from build123d import *

# Parameters (mm, degrees)
SKETCH1_W           = 8
SKETCH1_H           = 2
SKETCH1_W_2         = 2
SKETCH1_H_2         = 5
BOSS_EXTRUDE1_DEPTH = 2


with BuildPart() as part:
    # Sketch1 → Boss-Extrude1 (new body)
    with BuildSketch(Plane.XY):
        with BuildLine():
            Line((15.25, 3.5), (-15.25, 3.5))
            ThreePointArc((-15.25, 3.5), (-15.780330086, 3.280330086), (-16, 2.75))
            Line((-16, 2.75), (-16, -2.75))
            ThreePointArc((-16, -2.75), (-15.780330086, -3.280330086), (-15.25, -3.5))
            Line((-15.25, -3.5), (-3.5, -3.5))
            ThreePointArc((-3.5, -3.5), (-3.146446609, -3.646446609), (-3, -4))
            Line((-3, -4), (-3, -15.5))
            Line((-3, -15.5), (3, -15.5))
            Line((3, -15.5), (3, -4))
            ThreePointArc((3, -4), (3.146446609, -3.646446609), (3.5, -3.5))
            Line((3.5, -3.5), (15.25, -3.5))
            ThreePointArc((15.25, -3.5), (15.780330086, -3.280330086), (16, -2.75))
            Line((16, -2.75), (16, 2.75))
            ThreePointArc((16, 2.75), (15.780330086, 3.280330086), (15.25, 3.5))
        make_face()
        with Locations((-9, 0)):
            Rectangle(SKETCH1_W, SKETCH1_H, mode=Mode.SUBTRACT)
        with Locations((9, 0)):
            Rectangle(SKETCH1_W, SKETCH1_H, mode=Mode.SUBTRACT)
        with Locations((0, -11)):
            Rectangle(SKETCH1_W_2, SKETCH1_H_2, mode=Mode.SUBTRACT)
    extrude(amount=BOSS_EXTRUDE1_DEPTH)


solid = part.part
Here's how the part is built. I have some questions about the finished solid (model axes, mm). A direction names the side the tool comes from. Coordinates: 2 decimals unless noted, no trailing zeros. Order: outer loops, then holes, each group sorted by start corner. A loop starts at its lowest first (then second) coordinate and runs counter-clockwise, first axis right, second up. Notation, with made-up numbers: (-28, 2) - (-22, 2) arc R31 ccw to (-22, 35) - close; hole circle Ø5 at (-11, 52). An arc over 180 degrees is marked (long way). Use CSV: the item, a comma, the result in double quotes. Start each with the question number.
1. Suppose I cut it at B-B on z = 0.3. List the corners of the cut face in (x, y) for me, then the cut area to 3 significant figures.
2. Suppose I cut it at A-A on x = -9. List the corners of the cut face in (y, z) for me, then the cut area to 3 significant figures.
3. I'm going to push flat-ended pins straight in: pin 1 (1.5 mm diameter, centred on x = -9.5, y = 0, fed in from +Z); pin 2 (4 mm diameter, centred on x = 4, y = 0, fed in from -Z); pin 3 (0.6 mm diameter, centred on x = 8.5, z = 1, fed in from -Y). Where does each tip first touch, or does it pass through?
4. If we mould it in two halves opening along Y, with no side actions, what happens to faces 1 (the face through (0, 3.5, 1)), 2 (the face through (0, -3, 2)), 3 (the face through (-5, 0, 1))? For each: +Y half, -Y half, draft (parallel to the pull), parting line (faces both ways), or undercut.
5. For faces 4 (the face through (3, -10, 1)), 5 (the face through (-9, 1, 1)), 6 (the face through (-3, -10, 1)), which set-ups out of +Z, -Z, +X, -X, +Y, -Y let a thin tool reach every point of the face, with its end or its side?
6. Suppose I cut it at C-C on y = -14.25. List the corners of the cut face in (x, z) for me.
7. Suppose I cut it at D-D on x = 4. List the corners of the cut face in (y, z) for me.
8. Please list where these lines run through material, in increasing order: line 1 (Y direction, x = -9, z = 0.45); line 2 (X direction, y = -11, z = 1.35); line 3 (X direction, y = -4.25, z = 1.6). Write a range as from..to.
Output:
1,outline,"(-16, -2.75) arc R0.75 ccw to (-15.25, -3.5) - (-3.5, -3.5) arc R0.5 cw to (-3, -4) - (-3, -15.5) - (3, -15.5) - (3, -4) arc R0.5 cw to (3.5, -3.5) - (15.25, -3.5) arc R0.75 ccw to (16, -2.75) - (16, 2.75) arc R0.75 ccw to (15.25, 3.5) - (-15.25, 3.5) arc R0.75 ccw to (-16, 2.75) - close; hole (-13, -1) - (-5, -1) - (-5, 1) - (-13, 1) - close; hole (-1, -13.5) - (1, -13.5) - (1, -8.5) - (-1, -8.5) - close; hole (5, -1) - (13, -1) - (13, 1) - (5, 1) - close"
1,area,"254 mm2"
2,outline,"(-3.5, 0) - (-1, 0) - (-1, 2) - (-3.5, 2) - close; (1, 0) - (3.5, 0) - (3.5, 2) - (1, 2) - close"
2,area,"10.0 mm2"
3,pin 1,"passes through"
3,pin 2,"stops at z = 0"
3,pin 3,"stops at y = -3.5"
4,face 1,"+Y half"
4,face 2,"draft"
4,face 3,"undercut"
5,face 4,"+Z, -Z, +X, -Y"
5,face 5,"+Z, -Z"
5,face 6,"+Z, -Z, -X, -Y"
6,outline,"(-3, 0) - (3, 0) - (3, 2) - (-3, 2) - close"
7,outline,"(-3.5, 0) - (3.5, 0) - (3.5, 2) - (-3.5, 2) - close"
8,line 1,"y = -3.5..-1, 1..3.5"
8,line 2,"x = -3..-1, 1..3"
8,line 3,"x = -3..3"
